Autodesk Inventor part; units mm, degrees
ref_plane "YZ Plane" through (0, 0, 0) normal (1, 0, 0) x (0, 1, 0)
ref_plane "XZ Plane" through (0, 0, 0) normal (0, 1, 0) x (-1, 0, 0)
ref_plane "XY Plane" through (0, 0, 0) normal (0, 0, 1) x (1, 0, 0)
sketch "Sketch2" plane through (0, 0, 0) normal (0, 0, 1) x (1, 0, 0)
  line L0 (0, 0) -> (-44, 0)
  line L1 (-56, 12) -> (-56, 84)
  line L2 (-68, 96) -> (-112, 96)
  arc A0 (-56, 84) -> (-68, 96) centre (-68, 84) ccw
  arc A1 (-56, 12) -> (-44, 0) centre (-44, 12) ccw
  point P0 (-56, 0)
  point P1 (-56, 96)
  dimension "d0" = 56
  dimension "d1" = 96
  dimension "d2" = 56
  dimension "d3" = 12
sketch "Sketch3" plane through (0, 0, 0) normal (1, 0, 0) x (0, 1, 0)
  circle A0 centre (0, 0) radius 6
  dimension "d4" = 12
sweep "Sweep1" add profiles "Sketch3" path "Sketch2"
properties part number "handle"
Design review of the part built by this model. Coordinates are the model's own, in mm. A direction names the side the tool comes from. Give positions to 0.01 mm unless a question says otherwise; leave off trailing zeros. Order: outer loops, then holes, each group sorted by start corner. A loop starts at its lowest first (then second) coordinate and runs counter-clockwise, first axis right, second up. Notation, with made-up numbers: (39, -21) - (65, -21) arc R23 cw to (65, -5) - close; hole circle Ø5 at (37, 67). An arc over 180 degrees is marked (long way). Write item = value, one per line. Start each with the question number.
Q1. We need section B-B on y = 49. State the section outline as (x, z) points.
Q2. We need section A-A on z = 0. State the section outline as (x, y) points, plus the area to 3 significant figures.
Q3. We need section C-C on x = -75. State the section outline as (y, z) points.
Q4. Tool access review of faces 1 (the face through (-22, -6, 0)), 2 (the face through (-90, 90, 0)), 3 (the face through (-62, 49, 0)), 4 (the face through (0, 0, 0)), 5 (the face through (-112, 96, 0)): name each direction out of +Z, -Z, +X, -X, +Y, -Y from which nothing blocks a thin tool from reaching the whole face with its end or side.
Q5. Clearance check with flat-ended pins moving along their axes: pin 1 Ø1 at (y, z) = (7.5, -1.5) entering from +X; pin 2 Ø4 at (y, z) = (43.5, 0) entering from +X; pin 3 Ø2 at (y, z) = (54.5, 2) entering from +X. State where each tip first meets the part, or that it passes through.
Q6. To check wall thickness, follow L1, parallel to X at y = 70, z = -0.5; L2, parallel to Y at x = -90.5, z = 0.25; L3, parallel to X at y = 21.5, z = -3. State the ranges of each line that lie inside material, in increasing order. Write a range as from..to.
Working result:
q1.outline = circle Ø12 at (-56, 0)
q2.outline = (-112, 90) - (-68, 90) arc R6 cw to (-62, 84) - (-62, 12) arc R18 ccw to (-44, -6) - (0, -6) - (0, 6) - (-44, 6) arc R6 cw to (-50, 12) - (-50, 84) arc R18 ccw to (-68, 102) - (-112, 102) - close
q2.area = 2,370 mm²
q3.outline = circle Ø12 at (96, 0)
q4.face_1 = +X
q4.face_2 = -X
q4.face_3 = none
q4.face_4 = +Z, -Z, +X, +Y, -Y
q4.face_5 = +Z, -Z, -X, +Y, -Y
q5.pin_1 = -47.62
q5.pin_2 = -50
q5.pin_3 = -50.08
q6.L1 = -61.98..-50.02
q6.L2 = 90.01..101.99
q6.L3 = -61.2..-50.8
